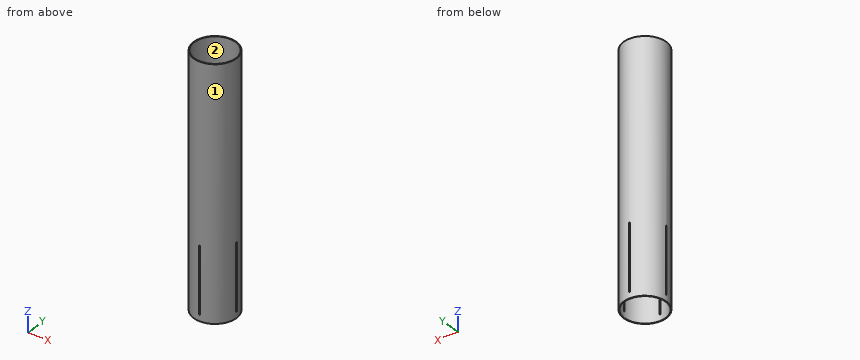
```python
from build123d import *

# Parameters (mm, degrees)
SKETCH1_R           = 65.405
SKETCH1_R_2         = 63.5
BOSS_EXTRUDE1_DEPTH = 381
SKETCH3_W           = 3.175
SKETCH3_H           = 203.2
CUT_EXTRUDE1_DEPTH  = 66.405
CIRPATTERN1_COUNT   = 4


with BuildPart() as part:
    # Sketch1 → Boss-Extrude1 (new body, symmetric)
    with BuildSketch(Plane.XY):
        Circle(SKETCH1_R)
        Circle(SKETCH1_R_2, mode=Mode.SUBTRACT)
    extrude(amount=BOSS_EXTRUDE1_DEPTH, both=True)

    # Sketch3 → Cut-Extrude1 (cut, through all)
    with BuildSketch(Plane(origin=(0, 0, 0), x_dir=(1, 0, 0), z_dir=(0, 1, 0))):
        with Locations((0, 260.35)):
            Rectangle(SKETCH3_W, SKETCH3_H)
    cut_extrude1 = extrude(amount=CUT_EXTRUDE1_DEPTH, mode=Mode.SUBTRACT)

    # CirPattern1: Cut-Extrude1 ×4 about axis
    cirpattern1_axis = Axis((0, 0, 0), (0, 0, 1))
    for i in range(1, CIRPATTERN1_COUNT):
        add(cut_extrude1.rotate(cirpattern1_axis, i * 360 / CIRPATTERN1_COUNT), mode=Mode.SUBTRACT)


solid = part.part
```
Model file for the job. Use its own axes, mm. Face numbers are marked on the shaded views. Round coordinates to 2 decimals unless told otherwise and drop trailing zeros. Order: outer loops, then holes, each group sorted by start corner. A loop starts at its lowest first (then second) coordinate and runs counter-clockwise, first axis right, second up. Notation, with made-up numbers: (32, 62) -> (36, 62) arc R26 cw to (36, 88) -> close; hole circle Ø4 at (37.5, 80). An arc over 180 degrees is marked (long way). Use one line per item in the form item = value.
Item 1: Flat gauge pins, fed straight in: pin 1 Ø8 at (x, z) = (25.5, 87) entering from +Y; pin 2 Ø8 at (y, z) = (-7.5, -97.5) entering from -X; pin 3 Ø10 at (x, z) = (20, 73) entering from +Y. Where does each tip first touch, or does it go through?
Returned:
pin_1 = 61.77
pin_2 = -65.31
pin_3 = 63.66
Item 2: Cut at A-A, the plane x = 40.5. Write the cut outline in (y, z), and give its area (3 significant figures).
Returned:
outline = (-51.36, -381) -> (-48.91, -381) -> (-48.91, 381) -> (-51.36, 381) -> close; (48.91, -381) -> (51.36, -381) -> (51.36, 381) -> (48.91, 381) -> close
area = 3,730 mm^2
Item 3: Cut at B-B, the plane y = 18.5. Write the cut outline in (x, z), and give its area (3 significant figures).
Returned:
outline = (-62.73, -381) -> (-60.75, -381) -> (-60.75, 381) -> (-62.73, 381) -> close; (60.75, -381) -> (62.73, -381) -> (62.73, 381) -> (60.75, 381) -> close
area = 3,030 mm^2
Item 4: Cut at C-C, the plane z = 75.5. Write the cut outline in (x, y) (3 decimals), and give its area (3 significant figures).
Returned:
outline = circle Ø130.81 at (0, 0); hole circle Ø127 at (0, 0)
area = 771 mm^2
Item 5: Pull direction X, two halves, no side cores. Call the marked faces 1 and 2: released by +X, released by -X, zero draft, split by the parting line, or undercut.
Returned:
face_1 = split by the parting line
face_2 = undercut
Item 6: Drill centre lines: line 1 (Y direction, x = 0, z = 98.5) (3 decimals); line 2 (X direction, y = -3.5, z = 286). Where is each one in solid material? Low to high.
Returned:
line_1 = -65.405 to -63.5, 63.5 to 65.405
line_2 = -65.31 to -63.4, 63.4 to 65.31
